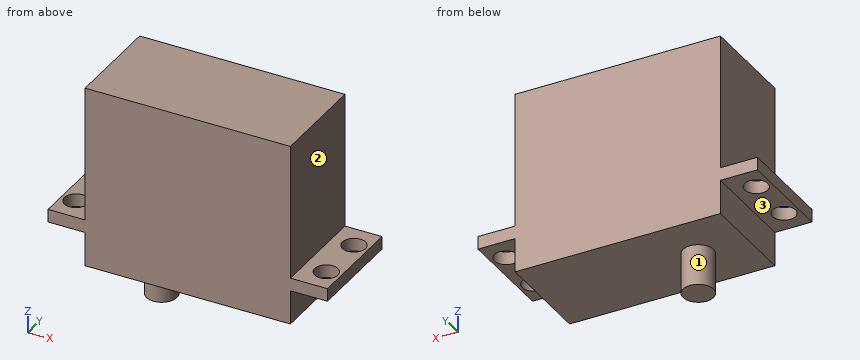
```python
from build123d import *

# Parameters (mm, degrees)
BOSS_EXTRUDE1_DEPTH = 19.685
SKETCH3_R           = 2.9845
BOSS_EXTRUDE2_DEPTH = 8.0264
CUT_EXTRUDE1_REACH  = 31.21
SKETCH4_R           = 2.286


with BuildPart() as part:
    # Sketch1 → Boss-Extrude1 (new body)
    with BuildSketch(Plane(origin=(0, 0, 0), x_dir=(1, 0, 0), z_dir=(0, 1, 0))):
        Polygon((0, 29.21), (0, 35.941), (40.386, 35.941), (40.386, 29.21), (47.6758, 29.21), (47.6758, 26.67), (40.386, 26.67), (40.386, 0), (0, 0), (0, 26.67), (-7.2898, 26.67), (-7.2898, 29.21), align=None)
    extrude(amount=BOSS_EXTRUDE1_DEPTH)

    # Sketch3 → Boss-Extrude2 (add)
    with BuildSketch(Plane(origin=(0, 0, -35.941), x_dir=(-1, 0, 0), z_dir=(0, 0, -1))):
        with Locations((-9.7155, 9.8425)):
            Circle(SKETCH3_R)
    extrude(amount=BOSS_EXTRUDE2_DEPTH)

    # Sketch4 → Cut-Extrude1 (cut, up to next)
    with BuildSketch(Plane(origin=(0, 0, -29.21), x_dir=(-1, 0, 0), z_dir=(0, 0, -1)), mode=Mode.PRIVATE) as cut_extrude1_sk1:
        with Locations((-44.8056, 14.859)):
            Circle(SKETCH4_R)
    cut_extrude1_tool1 = extrude(cut_extrude1_sk1.sketch, amount=-CUT_EXTRUDE1_REACH, mode=Mode.PRIVATE) & part.part
    add(cut_extrude1_tool1.solids().sort_by_distance((44.8056, 14.859, -29.21))[0], mode=Mode.SUBTRACT)
    # Sketch4 → Cut-Extrude1 (cut, up to next)
    with BuildSketch(Plane(origin=(0, 0, -29.21), x_dir=(-1, 0, 0), z_dir=(0, 0, -1)), mode=Mode.PRIVATE) as cut_extrude1_sk2:
        with Locations((-44.8056, 4.826)):
            Circle(SKETCH4_R)
    cut_extrude1_tool2 = extrude(cut_extrude1_sk2.sketch, amount=-CUT_EXTRUDE1_REACH, mode=Mode.PRIVATE) & part.part
    add(cut_extrude1_tool2.solids().sort_by_distance((44.8056, 4.826, -29.21))[0], mode=Mode.SUBTRACT)
    # Sketch4 → Cut-Extrude1 (cut, up to next)
    with BuildSketch(Plane(origin=(0, 0, -29.21), x_dir=(-1, 0, 0), z_dir=(0, 0, -1)), mode=Mode.PRIVATE) as cut_extrude1_sk3:
        with Locations((4.4196, 14.859)):
            Circle(SKETCH4_R)
    cut_extrude1_tool3 = extrude(cut_extrude1_sk3.sketch, amount=-CUT_EXTRUDE1_REACH, mode=Mode.PRIVATE) & part.part
    add(cut_extrude1_tool3.solids().sort_by_distance((-4.4196, 14.859, -29.21))[0], mode=Mode.SUBTRACT)
    # Sketch4 → Cut-Extrude1 (cut, up to next)
    with BuildSketch(Plane(origin=(0, 0, -29.21), x_dir=(-1, 0, 0), z_dir=(0, 0, -1)), mode=Mode.PRIVATE) as cut_extrude1_sk4:
        with Locations((4.4196, 4.826)):
            Circle(SKETCH4_R)
    cut_extrude1_tool4 = extrude(cut_extrude1_sk4.sketch, amount=-CUT_EXTRUDE1_REACH, mode=Mode.PRIVATE) & part.part
    add(cut_extrude1_tool4.solids().sort_by_distance((-4.4196, 4.826, -29.21))[0], mode=Mode.SUBTRACT)


solid = part.part
```
Geometry: final body of the model. Coordinates: model frame, mm. Face numbers are marked on the shaded views. A direction names the side the tool comes from. Round coordinates to 2 decimals unless told otherwise and drop trailing zeros. Loops run counter-clockwise (first coordinate to the right, second up) from the corner with the lowest first, then second, coordinate; pieces in that order, holes last. Notation, with made-up numbers: (35, 55) -> (56, 55) arc R19 ccw to (56, 74) -> close; hole circle Ø3 at (-1.5, -32). An arc over 180 degrees is marked (long way). Use one line per item in the form item = value.
Item 1: Access query for the marked faces 1, 2 and 3. Directions: +Z, -Z, +X, -X, +Y, -Y. A direction counts if a zero-diameter tool reaches every point of the face in a straight line with its end or side. Return the directions, or none.
Evaluation:
face_1 = -Z
face_2 = +Z, +X, +Y, -Y
face_3 = -Z, -X, +Y, -Y
Item 2: Material intervals for probe 1 along X at (y, z) = (18.25, -4.5); probe 2 along Z at (x, y) = (29, 16); probe 3 along Z at (x, y) = (41.5, 14), sorted ascending.
Evaluation:
probe_1 = 0 to 40.39
probe_2 = -35.94 to 0
probe_3 = -29.21 to -26.67
Item 3: Cut plane D-D on z = -16.5. Output: boundary loops of the cut face in (x, y) (3 decimals), then the cut area to 3 significant figures.
Evaluation:
outline = (0, 0) -> (40.386, 0) -> (40.386, 19.685) -> (0, 19.685) -> close
area = 795 mm2
Item 4: Cut plane A-A on y = 16.25. Output: boundary loops of the cut face in (x, z).
Evaluation:
outline = (-7.29, -29.21) -> (-6.23, -29.21) -> (-6.23, -26.67) -> (-7.29, -26.67) -> close; (-2.61, -29.21) -> (0, -29.21) -> (0, -35.94) -> (40.39, -35.94) -> (40.39, -29.21) -> (42.99, -29.21) -> (42.99, -26.67) -> (40.39, -26.67) -> (40.39, 0) -> (0, 0) -> (0, -26.67) -> (-2.61, -26.67) -> close; (46.62, -29.21) -> (47.68, -29.21) -> (47.68, -26.67) -> (46.62, -26.67) -> close
Item 5: Cut plane C-C on y = 10.5. Output: boundary loops of the cut face in (x, z), then the cut area to 3 significant figures.
Evaluation:
outline = (-7.29, -29.21) -> (0, -29.21) -> (0, -35.94) -> (6.8, -35.94) -> (6.8, -43.97) -> (12.63, -43.97) -> (12.63, -35.94) -> (40.39, -35.94) -> (40.39, -29.21) -> (47.68, -29.21) -> (47.68, -26.67) -> (40.39, -26.67) -> (40.39, 0) -> (0, 0) -> (0, -26.67) -> (-7.29, -26.67) -> close
area = 1,540 mm2
Item 6: Contact query for flat-ended pins moving along their axis: pin 1 Ø6 at (y, z) = (8, -19) entering from +X; pin 2 Ø6 at (x, y) = (-4.42, 14.86) entering from +Z; pin 3 Ø1.5 at (y, z) = (14.5, -17) entering from -X; pin 4 Ø4 at (x, y) = (-4.42, 4.83) entering from -Z. Output: stop coordinate, or through.
Evaluation:
pin_1 = 40.39
pin_2 = -26.67
pin_3 = 0
pin_4 = through
Item 7: Cut plane B-B on x = 8. Output: boundary loops of the cut face in (y, z) (3 decimals), then the cut area to 3 significant figures.
Evaluation:
outline = (0, -35.941) -> (7.4, -35.941) -> (7.4, -43.967) -> (12.285, -43.967) -> (12.285, -35.941) -> (19.685, -35.941) -> (19.685, 0) -> (0, 0) -> close
area = 747 mm2
